```python
from build123d import *

# Parameters (mm, degrees)
BOSS_EXTRUDE1_DEPTH = 3.5


with BuildPart() as part:
    # Sketch1 → Boss-Extrude1 (new body)
    with BuildSketch(Plane(origin=(0, 0, 0), x_dir=(1, 0, 0), z_dir=(0, 1, 0))):
        with BuildLine():
            Line((-4.5, -0.16424544), (-1.1, -0.16424544))
            Line((-1.1, -0.16424544), (-1.1, 0.945359747))
            ThreePointArc((-1.1, 0.945359747), (-1.37605082, 1.61180538), (-0.709605187, 1.33575456))
            Line((-0.709605187, 1.33575456), (0.709605187, 1.33575456))
            ThreePointArc((0.709605187, 1.33575456), (1.37605082, 1.61180538), (1.1, 0.945359747))
            Line((1.1, 0.945359747), (1.1, -0.16424544))
            Line((1.1, -0.16424544), (4.5, -0.16424544))
            Line((4.5, -0.16424544), (4.5, 2.74500456))
            Line((4.5, 2.74500456), (1, 2.74500456))
            Line((1, 2.74500456), (1, 7.24500456))
            Line((1, 7.24500456), (-1, 7.24500456))
            Line((-1, 7.24500456), (-1, 2.74500456))
            Line((-1, 2.74500456), (-4.5, 2.74500456))
            Line((-4.5, 2.74500456), (-4.5, -0.16424544))
        make_face()
    extrude(amount=BOSS_EXTRUDE1_DEPTH)


solid = part.part
```
Check sheet for the modelled part. Datum: model origin and axes. Units: mm. A direction names the side the tool comes from. Round coordinates to 2 decimals unless told otherwise and drop trailing zeros. Write each loop counter-clockwise with the first axis right and the second up, starting at its lowest first coordinate (ties: lowest second). Pieces come first, ordered by that corner, then holes. Notation, with made-up numbers: (27, -23) -> (43, -23) arc R8 cw to (43, -12) -> close; hole circle Ø11 at (78, 55.25). An arc over 180 degrees is marked (long way). One line per question, with ' | ' between items. Start each with the question number.
1. Sectioned sample at B-B, the plane x = 1.25. Record the cut outline in (y, z) (3 decimals), then the cut area to 3 significant figures.
2. Release check for a two-part mould opening along X. For faces 1 (the face through (0, 2, -1.336)), 2 (the face through (3, 2, -2.745)), 3 (the face through (1, 2, -5)), 4 (the face through (-1, 2, -5)) record: +X half, -X half, draft (parallel to the pull), parting line (faces both ways), or undercut.
3. Scan lines: line 1 along X through (y, z) = (1, -0.75); line 2 along Z through (x, y) = (-2, 2.9) (3 decimals); line 3 along X through (y, z) = (1.65, -5.5). Record each from-to range of solid material in increasing order. Write a range as from..to.
4. Sectioned sample at C-C, the plane x = -2.5. Record the cut outline in (y, z) (3 decimals), then the cut area to 3 significant figures.
5. Sectioned sample at D-D, the plane z = -3. Record the cut outline in (x, y).
6. Set-up check for faces 5 (the face through (0, 0, -3)), 6 (the face through (-1.1, 2, 0)), 7 (the face through (-3, 2, -2.745)): record each of +Z, -Z, +X, -X, +Y, -Y from which the full face is reachable in a straight line by a thin tool's end or side.
7. Depth check by flat-ended pin: pin 1 (1 mm diameter, centred on x = 3, y = 1, fed in from -Z) (3 decimals); pin 2 (1.6 mm diameter, centred on x = 0, y = 2, fed in from +Z); pin 3 (1.5 mm diameter, centred on y = 2.5, z = -4, fed in from -X). Enter the tip coordinate at first touch or a pass-through.
8. Sectioned sample at A-A, the plane y = 2. Record the cut outline in (x, z) (3 decimals), then the cut area to 3 significant figures.
Taken from the geometry:
1) outline: (0, -2.745) -> (3.5, -2.745) -> (3.5, -1.696) -> (0, -1.696) -> close; (0, -0.975) -> (3.5, -0.975) -> (3.5, 0.164) -> (0, 0.164) -> close | area: 7.66 mm^2
2) face 1: undercut | face 2: draft | face 3: +X half | face 4: -X half
3) line 1: x = -4.5..-1.1, 1.1..4.5 | line 2: z = -2.745..0.164 | line 3: x = -1..1
4) outline: (0, -2.745) -> (3.5, -2.745) -> (3.5, 0.164) -> (0, 0.164) -> close | area: 10.2 mm^2
5) outline: (-1, 0) -> (1, 0) -> (1, 3.5) -> (-1, 3.5) -> close
6) face 5: +Z, -Z, +X, -X, -Y | face 6: +Z, +Y, -Y | face 7: -Z, -X, +Y, -Y
7) pin 1: stops at z = -2.745 | pin 2: stops at z = -1.34 | pin 3: stops at x = -1
8) outline: (-4.5, -2.745) -> (-1, -2.745) -> (-1, -7.245) -> (1, -7.245) -> (1, -2.745) -> (4.5, -2.745) -> (4.5, 0.164) -> (1.1, 0.164) -> (1.1, -0.945) arc R0.39 cw (long way) to (0.71, -1.336) -> (-0.71, -1.336) arc R0.39 cw (long way) to (-1.1, -0.945) -> (-1.1, 0.164) -> (-4.5, 0.164) -> close | area: 31.2 mm^2
